Part model, mm, in its own coordinate system. A direction names the side the tool comes from. Coordinates: 2 decimals unless noted, no trailing zeros. Order: outer loops, then holes, each group sorted by start corner. A loop starts at its lowest first (then second) coordinate and runs counter-clockwise, first axis right, second up. Notation, with made-up numbers: M 51.25,16 L 61.25,16 A11 ccw 61.25,35 Z; hole C -13,13.5 d7. An arc over 180 degrees is marked long. Write item = value, one per line. Start each with the question number.
from build123d import *

# Parameters (mm, degrees)
ESQUISSE1_R             = 13.75
BOSS_EXTRU_1_DEPTH      = 9
ENL_V_START             = -1
ESQUISSE2_OUTSIDE_W     = 37.484
ESQUISSE2_OUTSIDE_H     = 37.484
ESQUISSE2_OUTSIDE_R     = 7.75
ENL_V_MAT_EXTRU_1_DEPTH = 7
ENL_V_MAT_EXTRU_2_REACH = 11
ESQUISSE3_R             = 7.05
ENL_V_MAT_EXTRU_3_REACH = 11
ESQUISSE4_R             = 0.5
ESQUISSE5_W             = 2
ESQUISSE5_H             = 15.584719065
ENL_V_MAT_EXTRU_4_DEPTH = 0.7


with BuildPart() as part:
    # Esquisse1 → Boss.-Extru.1 (new body)
    with BuildSketch(Plane(origin=(0, 0, 0), x_dir=(1, 0, 0), z_dir=(0, 1, 0))):
        with Locations(Location((0, 0, 0), (0, 0, 270))):  # turned: the seam where the file's is
            Circle(ESQUISSE1_R)
    extrude(amount=BOSS_EXTRU_1_DEPTH)

    # Esquisse2 outside → Enlèv. mat.-Extru.1 (cut)
    with BuildSketch(Plane(origin=(0, 9, 0), x_dir=(-1, 0, 0), z_dir=(0, 1, 0)).offset(ENL_V_START)):
        Rectangle(ESQUISSE2_OUTSIDE_W, ESQUISSE2_OUTSIDE_H)
        with Locations(Location((0, 0, 0), (0, 0, 90))):  # turned: the seam where the file's is
            Circle(ESQUISSE2_OUTSIDE_R, mode=Mode.SUBTRACT)
    extrude(amount=-ENL_V_MAT_EXTRU_1_DEPTH, mode=Mode.SUBTRACT)

    # Esquisse3 → Enlèv. mat.-Extru.2 (cut, up to next)
    with BuildSketch(Plane(origin=(0, 9, 0), x_dir=(-1, 0, 0), z_dir=(0, 1, 0)), mode=Mode.PRIVATE) as enl_v_mat_extru_2_sk1:
        with Locations(Location((0, 0, 0), (0, 0, 90))):  # turned: the seam where the file's is
            Circle(ESQUISSE3_R)
    enl_v_mat_extru_2_tool1 = extrude(enl_v_mat_extru_2_sk1.sketch, amount=-ENL_V_MAT_EXTRU_2_REACH, mode=Mode.PRIVATE) & part.part
    add(enl_v_mat_extru_2_tool1.solids().sort_by_distance((0, 9, 0))[0], mode=Mode.SUBTRACT)

    # Esquisse4 → Enlèv. mat.-Extru.3 (cut, up to next)
    with BuildSketch(Plane(origin=(0, 9, 0), x_dir=(-1, 0, 0), z_dir=(0, 1, 0)), mode=Mode.PRIVATE) as enl_v_mat_extru_3_sk1:
        with Locations(Location((0, 8.256283794, 0), (0, 0, 90))):  # turned: the seam where the file's is
            Circle(ESQUISSE4_R)
    enl_v_mat_extru_3_tool1 = extrude(enl_v_mat_extru_3_sk1.sketch, amount=-ENL_V_MAT_EXTRU_3_REACH, mode=Mode.PRIVATE) & part.part
    add(enl_v_mat_extru_3_tool1.solids().sort_by_distance((0, 9, 8.256284))[0], mode=Mode.SUBTRACT)
    # Esquisse4 → Enlèv. mat.-Extru.3 (cut, up to next)
    with BuildSketch(Plane(origin=(0, 9, 0), x_dir=(-1, 0, 0), z_dir=(0, 1, 0)), mode=Mode.PRIVATE) as enl_v_mat_extru_3_sk2:
        with Locations(Location((0, 12.75, 0), (0, 0, 90))):  # turned: the seam where the file's is
            Circle(ESQUISSE4_R)
    enl_v_mat_extru_3_tool2 = extrude(enl_v_mat_extru_3_sk2.sketch, amount=-ENL_V_MAT_EXTRU_3_REACH, mode=Mode.PRIVATE) & part.part
    add(enl_v_mat_extru_3_tool2.solids().sort_by_distance((0, 9, 12.75))[0], mode=Mode.SUBTRACT)

    # Esquisse5 → Enlèv. mat.-Extru.4 (cut)
    with BuildSketch(Plane(origin=(0, 9, 0), x_dir=(-1, 0, 0), z_dir=(0, 1, 0))):
        with Locations((0, 7.792359533)):
            Rectangle(ESQUISSE5_W, ESQUISSE5_H)
    extrude(amount=-ENL_V_MAT_EXTRU_4_DEPTH, mode=Mode.SUBTRACT)


solid = part.part
Item 1: Cut at B-B, the plane z = -11. Write the cut outline in (x, y), and give its area (3 significant figures).
Item 2: Cut at D-D, the plane y = 4. Write the cut outline in (x, z).
Item 3: Pull direction Z, two halves, no side cores. Call faces 1 (the flat face through (-6, 9, 6)), 2 (the cylindrical face through (-12.2, 8.49, 6.34)), 3 (the cylindrical face through (0.02, 8.15, 12.25)): pulls with the +Z half, pulls with the -Z half, needs draft (parallel to the pull), parting line crosses it, or undercut.
Item 4: Flat gauge pins, fed straight in: pin 1 (0.8 mm diameter, centred on y = 8.5, z = 12, fed in from +X); pin 2 (1.6 mm diameter, centred on x = -0.5, z = 10.5, fed in from +Y); pin 3 (1 mm diameter, centred on x = -4.5, y = 4.5, fed in from +Z). Where does each tip first touch, or does it go through?
Item 5: Wall check: line 1 along Y through (x, z) = (8.5, -2.5); line 2 along X through (y, z) = (5.75, 0); line 3 along X through (y, z) = (4.5, -4.75). Give the ranges that are in metal, low to high. Write a range as [from, to].
Item 6: 3-axis set-ups, long thin cutter, end or side, ignore diameter. For faces 4 (the flat face through (0, 8.3, 10)), 5 (the cylindrical face through (-0.19, 8.15, 8.72)), 6 (the flat face through (-6, 1, -6)): which of +Z, -Z, +X, -X, +Y, -Y reach the whole face in a straight line?
Item 7: Cut at A-A, the plane x = 0. Count the separate pieces of the cut face and the enclosed holes in it, and give its area (3 significant figures).
Item 8: Cut at C-C, the plane x = 2.75. Write the cut outline in (y, z).
Filled sheet:
q1.outline = M -8.25,0 L 8.25,0 L 8.25,1 L -8.25,1 Z; M -8.25,8 L 8.25,8 L 8.25,9 L -8.25,9 Z
q1.area = 33.0 mm2
q2.outline = C 0,0 d15.5; hole C 0,0 d14.1
q3.face_1 = needs draft
q3.face_2 = parting line crosses it
q3.face_3 = undercut
q4.pin_1 = 7.38
q4.pin_2 = 9
q4.pin_3 = 6.64
q5.line_1 = [0, 1], [8, 9]
q5.line_2 = [-7.75, -7.05], [7.05, 7.75]
q5.line_3 = [-6.12, -5.21], [5.21, 6.12]
q6.face_4 = +Z, +Y
q6.face_5 = +Y
q6.face_6 = none
q7.separate_pieces = 4
q7.enclosed_holes = 0
q7.area = 31.3 mm2
q8.outline = M 0,-13.47 L 1,-13.47 L 1,-7.25 L 8,-7.25 L 8,-13.47 L 9,-13.47 L 9,-6.49 L 0,-6.49 Z; M 0,6.49 L 9,6.49 L 9,13.47 L 8,13.47 L 8,7.25 L 1,7.25 L 1,13.47 L 0,13.47 Z
